For this review, take the finished solid that the model builds, in its own axes (mm). Face numbers are marked on the shaded views. A direction names the side the tool comes from. Round coordinates to 2 decimals unless told otherwise and drop trailing zeros. Loops run counter-clockwise (first coordinate to the right, second up) from the corner with the lowest first, then second, coordinate; pieces in that order, holes last.
1) Take a section at B-B (y = 6.25). State the section outline as (x, z) points, then the cut area to 3 significant figures.
2) Tool access review of the marked faces 1, 2, 3 and 4: name each direction out of +Z, -Z, +X, -X, +Y, -Y from which nothing blocks a thin tool from reaching the whole face with its end or side.
3) Take a section at A-A (x = 8.5). State the section outline as (y, z) points, then the cut area to 3 significant figures.
4) Wall thickness on L1, parallel to Y at x = 13.4, z = -5.5; L2, parallel to Z at x = 13, y = 4; L3, parallel to X at y = 2.5, z = 6.25: over which ranges is each line inside the solid? List them lowest first.
5) Mouldability with a two-part tool opening along Z and no side actions: class the marked faces 5, 6 and 7 as pulls with the +Z half, pulls with the -Z half, needs draft (parallel to the pull), parting line crosses it, or undercut.
6) Insertion check: pin 1 (3 mm diameter, centred on x = -13, z = 3.5, fed in from -Y); pin 2 (2 mm diameter, centred on y = 3.5, z = 5.5, fed in from +X). Each pin has a flat end and moves straight along its axis. Give the tip position at first contact, or say it passes through.
```python
from build123d import *

# Parameters (mm, degrees)
BOSS_EXTRUDE1_DEPTH = 7
FILLET1_R           = 2
SKETCH2_R           = 1.5
SKETCH2_R_2         = 1.1
BOSS_EXTRUDE2_DEPTH = 4
SKETCH3_R           = 1.5
SKETCH3_R_2         = 1.1
SKETCH3_W           = 4.5
SKETCH3_H           = 1.5
BOSS_EXTRUDE3_DEPTH = 4


with BuildPart() as part:
    # Sketch1 → Boss-Extrude1 (new body)
    with BuildSketch(Plane(origin=(0, 0, 0), x_dir=(1, 0, 0), z_dir=(0, 1, 0))):
        with BuildLine():
            Line((10, -9), (-10, -9))
            ThreePointArc((-10, -9), (-11.414213562, -8.414213562), (-12, -7))
            Line((-12, -7), (-12, 7))
            ThreePointArc((-12, 7), (-11.414213562, 8.414213562), (-10, 9))
            Line((-10, 9), (10, 9))
            ThreePointArc((10, 9), (11.414213562, 8.414213562), (12, 7))
            Line((12, 7), (12, -7))
            ThreePointArc((12, -7), (11.414213562, -8.414213562), (10, -9))
        make_face()
    extrude(amount=BOSS_EXTRUDE1_DEPTH)

    # Fillet1
    fillet1_edges = [part.edges().sort_by_distance(p)[0] for p in [
        (11.414213562, 7, 8.414213562),
        (0, 0, 9),
        (-11.414213562, 0, 8.414213562),
        (12, 7, 0),
        (11.414213562, 7, -8.414213562),
        (0, 7, -9),
        (-11.414213562, 7, -8.414213562),
        (-12, 7, 0),
        (-11.414213562, 7, 8.414213562),
        (0, 7, 9),
        (-12, 0, 0),
        (-11.414213562, 0, -8.414213562),
        (0, 0, -9),
        (11.414213562, 0, -8.414213562),
        (12, 0, 0),
        (11.414213562, 0, 8.414213562),
    ]]
    fillet(fillet1_edges, radius=FILLET1_R)

    # Sketch2 → Boss-Extrude2 (add)
    with BuildSketch(Plane(origin=(12, 0, 0), x_dir=(0, 0, -1), z_dir=(1, 0, 0))):
        with Locations((0, 3.5)):
            Circle(SKETCH2_R)
        with Locations((0, 3.5)):
            Circle(SKETCH2_R_2, mode=Mode.SUBTRACT)
        with Locations((-5.5, 3.5)):
            Circle(SKETCH2_R)
        with Locations((-5.5, 3.5)):
            Circle(SKETCH2_R_2, mode=Mode.SUBTRACT)
        with Locations((5.5, 3.5)):
            Circle(SKETCH2_R)
        with Locations((5.5, 3.5)):
            Circle(SKETCH2_R_2, mode=Mode.SUBTRACT)
    extrude(amount=BOSS_EXTRUDE2_DEPTH)

    # Sketch3 → Boss-Extrude3 (add)
    with BuildSketch(Plane.ZY.offset(12)):
        with Locations((-5.5, 3.5)):
            Circle(SKETCH3_R)
        with Locations((-5.5, 3.5)):
            Circle(SKETCH3_R_2, mode=Mode.SUBTRACT)
        with Locations((-1.1, 3.5)):
            Circle(SKETCH3_R)
        with Locations((-1.1, 3.5)):
            Circle(SKETCH3_R_2, mode=Mode.SUBTRACT)
        with Locations((4.031327063, 3.5)):
            Rectangle(SKETCH3_W, SKETCH3_H)
    extrude(amount=BOSS_EXTRUDE3_DEPTH)


solid = part.part
```
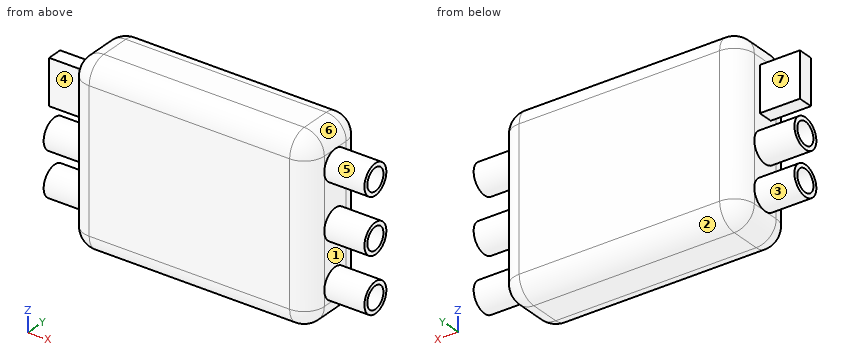
Response:
1. outline: (-11.56, -7) arc R1.56 ccw to (-10, -8.56) - (10, -8.56) arc R1.56 ccw to (11.56, -7) - (11.56, 7) arc R1.56 ccw to (10, 8.56) - (-10, 8.56) arc R1.56 ccw to (-11.56, 7) - close
1. area: 394 mm2
2. face 1: +X
2. face 2: -Z, +X, -X, +Y
2. face 3: -X
2. face 4: +Z, -X, -Y
3. outline: (0, -7) arc R2 ccw to (2, -9) - (5, -9) arc R2 ccw to (7, -7) - (7, 7) arc R2 ccw to (5, 9) - (2, 9) arc R2 ccw to (0, 7) - close
3. area: 123 mm2
4. L1: y = 2 to 2.4, 4.6 to 5
4. L2: z = -6.91 to -6.48, -4.52 to -4.09, -1.41 to -0.98, 0.98 to 1.41, 4.09 to 4.52, 6.48 to 6.91
4. L3: x = -12 to 16
5. face 5: undercut
5. face 6: pulls with the +Z half
5. face 7: needs draft
6. pin 1: stops at y = 0.68
6. pin 2: stops at x = 12
